Read the model definition and answer for the solid it produces. Units are mm, in the model's axes. Face numbers are marked on the shaded views. A direction names the side the tool comes from. Round coordinates to 2 decimals unless told otherwise and drop trailing zeros. Write each loop counter-clockwise with the first axis right and the second up, starting at its lowest first coordinate (ties: lowest second). Pieces come first, ordered by that corner, then holes. Notation, with made-up numbers: (63.5, -1.75) - (118.5, -1.75) arc R13 cw to (118.5, 14.25) - close; hole circle Ø9 at (-13, 77). An arc over 180 degrees is marked (long way). Answer as CSV lines item,"result". Start each with the question number.
1) Find section D-D on z = 5. Determine the outline of the cut face in (x, y).
2) Find section A-A on z = 39.5. Determine the outline of the cut face in (x, y), then the cut area to 3 significant figures.
3) Consider line 1 along Z through (x, y) = (0, 0); line 2 along Z through (x, y) = (1.75, -3.75); line 3 along Z through (x, y) = (5, 0). Determine where each line is inside the solid, lowest interval first.
4) Which of the six approach directions +Z, -Z, +X, -X, +Y, -Y give full straight-line access (tool end or side, diameter ignored) to the marked faces 1, 2 and 3?
5) Find section B-B on y = 0. Determine the outline of the cut face in (x, z).
6) Find section C-C on z = -7. Determine the outline of the cut face in (x, y), then the cut area to 3 significant figures.
7) For a pull along Y with two mould halves and no side action, classify the marked faces 4, 5, 6 and 7 as +Y half, -Y half, draft (parallel to the pull), parting line (faces both ways), or undercut.
8) Each of these flat-tipped pins is pushed along its axis until it touches: pin 1 (2.5 mm diameter, centred on y = 0, z = 39.5, fed in from +X); pin 2 (1.2 mm diameter, centred on x = 0.5, z = 40, fed in from -Y); pin 3 (8 mm diameter, centred on x = 0, y = 0, fed in from -Z); pin 4 (2 mm diameter, centred on x = 7, y = 2, fed in from +Z). Where does it stop, or does it pass through?
from build123d import *

# Parameters (mm, degrees)
SKETCH1_W           = 19
SKETCH1_H           = 22.5
BOSS_EXTRUDE1_DEPTH = 37
BOSS_EXTRUDE2_DEPTH = 11
FILLET1_R           = 5
SKETCH3_R           = 1.6
CUT_EXTRUDE1_DEPTH  = 44.087846314
SKETCH4_W           = 2.5
SKETCH4_H           = 5
BOSS_EXTRUDE3_DEPTH = 5
FILLET2_R           = 0.5
SKETCH5_R           = 1.5
CUT_EXTRUDE2_DEPTH  = 5
SKETCH6_R           = 2.8
CUT_EXTRUDE3_DEPTH  = 48.450632264
CUT_EXTRUDE4_DEPTH  = 11
SKETCH8_R           = 3
CUT_EXTRUDE5_DEPTH  = 2


with BuildPart() as part:
    # Sketch1 → Boss-Extrude1 (new body)
    with BuildSketch(Plane.XY):
        Rectangle(SKETCH1_W, SKETCH1_H)
    extrude(amount=BOSS_EXTRUDE1_DEPTH)

    # Sketch2 → Boss-Extrude2 (add)
    with BuildSketch(Plane(origin=(0, 0, 0), x_dir=(-1, 0, 0), z_dir=(0, 0, -1))):
        with BuildLine():
            Line((9.5, 6.025985397), (9.5, -6.025985397))
            ThreePointArc((9.5, -6.025985397), (0, -11.25), (-9.5, -6.025985397))
            Line((-9.5, -6.025985397), (-9.5, 6.025985397))
            ThreePointArc((-9.5, 6.025985397), (0, 11.25), (9.5, 6.025985397))
        make_face()
    extrude(amount=BOSS_EXTRUDE2_DEPTH)

    # Fillet1
    fillet1_edges = [part.edges().sort_by_distance(p)[0] for p in [
        (0, 11.25, 37),
        (0, -11.25, 37),
    ]]
    fillet(fillet1_edges, radius=FILLET1_R)

    # Sketch3 → Cut-Extrude1 (cut, through all)
    with BuildSketch(Plane(origin=(9.5, 0, 0), x_dir=(0, 0, -1), z_dir=(1, 0, 0))):
        with Locations(Location((-5, 8.75, 0), (0, 0, 90))):
            Circle(SKETCH3_R)
        with Locations(Location((-5, -8.75, 0), (0, 0, 90))):
            Circle(SKETCH3_R)
    extrude(amount=-CUT_EXTRUDE1_DEPTH, mode=Mode.SUBTRACT)

    # Sketch4 → Boss-Extrude3 (add)
    with BuildSketch(Plane.XY.offset(37)):
        Rectangle(SKETCH4_W, SKETCH4_H)
    extrude(amount=BOSS_EXTRUDE3_DEPTH)

    # Fillet2
    fillet2_edges = [part.edges().sort_by_distance(p)[0] for p in [
        (-9.5, 0, 37),
        (9.5, 0, 37),
        (9.5, 11.25, 16),
        (9.5, -11.25, 16),
        (9.5, 9.785533906, 35.535533906),
        (9.5, -9.785533906, 35.535533906),
        (-9.5, -11.25, 16),
        (-9.5, 11.25, 16),
        (-9.5, 9.785533906, 35.535533906),
        (-9.5, -9.785533906, 35.535533906),
        (0, -2.5, 42),
        (0, 2.5, 42),
    ]]
    fillet(fillet2_edges, radius=FILLET2_R)

    # Sketch5 → Cut-Extrude2 (cut)
    with BuildSketch(Plane(origin=(1.25, 0, 0), x_dir=(0, 0, -1), z_dir=(1, 0, 0))):
        with Locations(Location((-39.5, 0, 0), (0, 0, 90))):
            Circle(SKETCH5_R)
    extrude(amount=-CUT_EXTRUDE2_DEPTH, mode=Mode.SUBTRACT)

    # Sketch6 → Cut-Extrude3 (cut, through all)
    with BuildSketch(Plane(origin=(9.5, 0, 0), x_dir=(0, 0, -1), z_dir=(1, 0, 0))):
        with Locations(Location((-25.5, 0, 0), (0, 0, 90))):
            Circle(SKETCH6_R)
    extrude(amount=-CUT_EXTRUDE3_DEPTH, mode=Mode.SUBTRACT)

    # Sketch7 → Cut-Extrude4 (cut)
    with BuildSketch(Plane(origin=(0, 0, -11), x_dir=(-1, 0, 0), z_dir=(0, 0, -1))):
        with BuildLine():
            Line((-8.3, 5.666789214), (-8.3, -5.666789214))
            ThreePointArc((-8.3, -5.666789214), (0, -10.05), (8.3, -5.666789214))
            Line((8.3, -5.666789214), (8.3, 5.666789214))
            ThreePointArc((8.3, 5.666789214), (0, 10.05), (-8.3, 5.666789214))
        make_face()
    extrude(amount=-CUT_EXTRUDE4_DEPTH, mode=Mode.SUBTRACT)

    # Sketch8 → Cut-Extrude5 (cut)
    with BuildSketch(Plane(origin=(0, 0, 0), x_dir=(-1, 0, 0), z_dir=(0, 0, -1))):
        Circle(SKETCH8_R)
    extrude(amount=-CUT_EXTRUDE5_DEPTH, mode=Mode.SUBTRACT)


solid = part.part
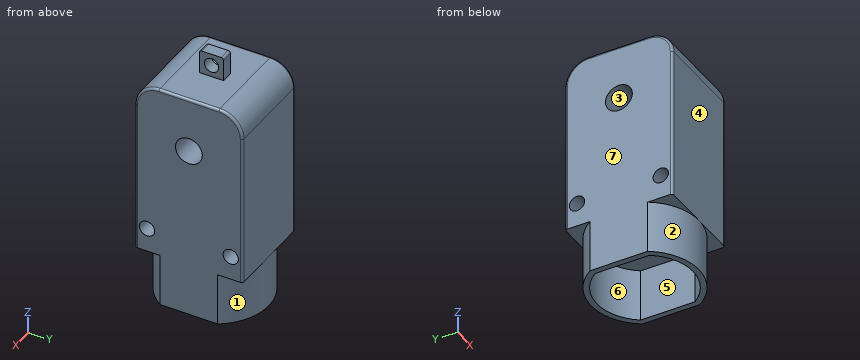
Check values:
1,outline,"(-9.5, -10.75) arc R0.5 ccw to (-9, -11.25) - (9, -11.25) arc R0.5 ccw to (9.5, -10.75) - (9.5, -10.35) - (-9.5, -10.35) - close; (-9.5, -7.15) - (9.5, -7.15) - (9.5, 7.15) - (-9.5, 7.15) - close; (-9.5, 10.35) - (9.5, 10.35) - (9.5, 10.75) arc R0.5 ccw to (9, 11.25) - (-9, 11.25) arc R0.5 ccw to (-9.5, 10.75) - close"
2,outline,"(-1.25, -2.5) - (1.25, -2.5) - (1.25, -1.5) - (-1.25, -1.5) - close; (-1.25, 1.5) - (1.25, 1.5) - (1.25, 2.5) - (-1.25, 2.5) - close"
2,area,"5.00 mm^2"
3,line 1,"z = 2 to 22.7, 28.3 to 38, 41 to 42"
3,line 2,"z = 0 to 37"
3,line 3,"z = 0 to 22.7, 28.3 to 37"
4,face 1,"-Z, +Y"
4,face 2,"-Z, -Y"
4,face 3,"+X, -X"
5,outline,"(-9.5, -11) - (-8.3, -11) - (-8.3, 0) - (-3, 0) - (-3, 2) - (3, 2) - (3, 0) - (8.3, 0) - (8.3, -11) - (9.5, -11) - (9.5, 22.7) - (-9.5, 22.7) - close; (-9.5, 28.3) - (9.5, 28.3) - (9.5, 36.5) arc R0.5 ccw to (9, 37) - (1.25, 37) - (1.25, 38) - (-1.25, 38) - (-1.25, 37) - (-9, 37) arc R0.5 ccw to (-9.5, 36.5) - close; (-1.25, 41) - (1.25, 41) - (1.25, 42) - (-1.25, 42) - close"
6,outline,"(-9.5, -6.03) arc R11.25 ccw to (9.5, -6.03) - (9.5, 6.03) arc R11.25 ccw to (-9.5, 6.03) - close; hole (-8.3, -5.67) arc R10.05 ccw to (8.3, -5.67) - (8.3, 5.67) arc R10.05 ccw to (-8.3, 5.67) - close"
6,area,"78.7 mm^2"
7,face 4,"-Y half"
7,face 5,"undercut"
7,face 6,"undercut"
7,face 7,"draft"
8,pin 1,"passes through"
8,pin 2,"stops at y = -2.5"
8,pin 3,"stops at z = 0"
8,pin 4,"stops at z = 37"
